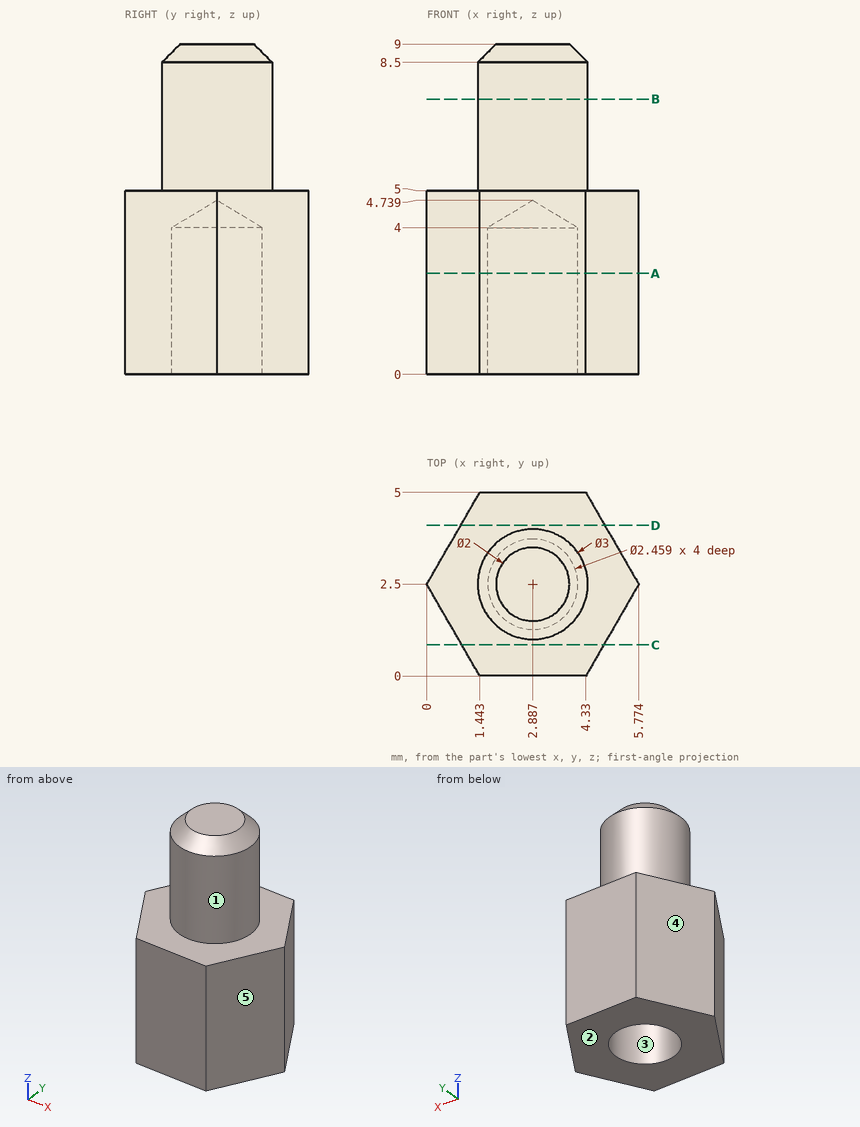
For this review, use the dimensioned drawing (mm, ordinates from the lowest corner) and the shaded views. A direction names the side the tool comes from. Round coordinates to 2 decimals unless told otherwise and drop trailing zeros. Write each loop counter-clockwise with the first axis right and the second up, starting at its lowest first coordinate (ties: lowest second). Pieces come first, ordered by that corner, then holes. Notation, with made-up numbers: (-32, 40) - (-12, 40) arc R26 cw to (-12, 63) - close; hole circle Ø8 at (-19, 41.5). An arc over 180 degrees is marked (long way). Answer as CSV lines item,"result". Start each with the question number.
(1) To check wall thickness, follow line 1 (Y direction, x = 2.8, z = 1.25); line 2 (Z direction, x = 4.4, y = 3.6); line 3 (Y direction, x = 2.45, z = 1.5). State the ranges of each line that lie inside material, in increasing order.
(2) For the marked faces 1 and 2, list the 3-axis set-ups (+Z, -Z, +X, -X, +Y, -Y) from which the entire face can be reached by the end or side of a thin tool; tool diameter is ignored.
(3) Draft analysis for pull direction X (two halves, no side actions). For the marked faces 3, 4 and 5, state which applies: pulls with the +X half, pulls with the -X half, needs draft (parallel to the pull), parting line crosses it, or undercut.
(4) We need section B-B on z = 7.5. State the section outline as (x, y) points.
(5) We need section A-A on z = 2.75. State the section outline as (x, y) points.
(6) We need section D-D on y = 4.1. State the section outline as (x, z) points.
(7) We need section C-C on y = 0.85. State the section outline as (x, z) points.
(8) For pin 1 Ø2 at (y, z) = (3.5, 8) entering from +X; pin 2 Ø1 at (y, z) = (4, 4) entering from +X; pin 3 Ø2 at (x, y) = (2.89, 2.5) entering from -Z (1 decimal), all flat-tipped, find the tip position at first contact; note any pin that passes through.
Worked answers:
1,line 1,"0 to 1.27, 3.73 to 5"
1,line 2,"0 to 5"
1,line 3,"0 to 1.35, 3.65 to 5"
2,face 1,"+Z"
2,face 2,"-Z, +X, -X, +Y, -Y"
3,face 3,"undercut"
3,face 4,"pulls with the -X half"
3,face 5,"pulls with the +X half"
4,outline,"circle Ø3 at (2.89, 2.5)"
5,outline,"(0, 2.5) - (1.44, 0) - (4.33, 0) - (5.77, 2.5) - (4.33, 5) - (1.44, 5) - close; hole circle Ø2.46 at (2.89, 2.5)"
6,outline,"(0.92, 0) - (4.85, 0) - (4.85, 5) - (0.92, 5) - close"
7,outline,"(0.95, 0) - (4.82, 0) - (4.82, 5) - (0.95, 5) - close"
8,pin 1,"x = 4.39"
8,pin 2,"x = 5.2"
8,pin 3,"z = 4.1"
